Autodesk Inventor part; units mm, degrees
ref_plane "YZ Plane" through (0, 0, 0) normal (1, 0, 0) x (0, 1, 0)
ref_plane "XZ Plane" through (0, 0, 0) normal (0, 1, 0) x (-1, 0, 0)
ref_plane "XY Plane" through (0, 0, 0) normal (0, 0, 1) x (1, 0, 0)
sketch "Sketch1" plane through (0, 0, 0) normal (0, 0, 1) x (1, 0, 0)
  line L0 (0, 0) -> (0, 50)
  line L1 (0, 50) -> (40, 50)
  line L2 (40, 50) -> (40, 20)
  line L3 (40, 20) -> (200, 20)
  line L4 (200, 20) -> (200, 0)
  line L5 (200, 0) -> (0, 0)
  line L6 (20, 50) -> (20, -1.8826)
  line L7 (20, -1.8826) -> (20, 0)
  circle A0 centre (20, 24.0587) radius 10
  dimension "d0" = 200
  dimension "d1" = 50
  dimension "d2" = 40
  dimension "d3" = 20
  dimension "d4" = 20
extrude "Extrusion1" add sketch "Sketch1" along normal blind 140 contours L0 L1 L6 A0 L5 | L6 A0 L1 L2 L3 L4 L5
fillet "Fillet1" radius 15 4 edges at (0, 50, 70) (40, 50, 70) (40, 20, 70) (0, 0, 70)
fillet "Fillet2" radius 20 2 edges at (200, 10, 140) (200, 10, 0)
fillet "Fillet3" radius 4 22 edges at (4.3933, 45.6067, 0) (0, 25, 0) (4.3933, 4.3933, 0) (97.4998, 0, 0) (194.1421, 0, 5.8579) (200, 0, 70) (194.1421, 0, 134.1421) (97.4998, 0, 140) (4.3933, 4.3933, 140) (0, 25, 140) (4.3933, 45.6067, 140) (20, 50, 140) (35.6067, 45.6067, 140) (40, 35, 140) (117.4998, 20, 140) (194.1421, 20, 134.1421) (200, 20, 70) (194.1421, 20, 5.8579) (117.4998, 20, 0) (40, 35, 0) (35.6067, 45.6067, 0) (20, 50, 0)
properties part number "foot rest EG26"
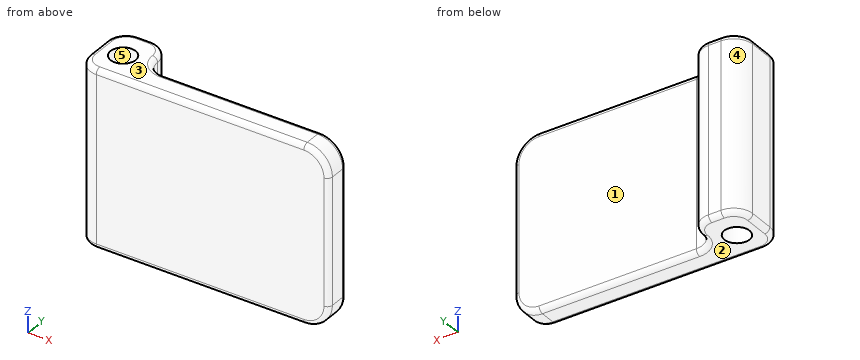
Could you check a few things on this model? Use its own coordinates, in mm. Face numbers are marked on the shaded views. A direction names the side the tool comes from. Coordinates: 2 decimals unless noted, no trailing zeros. Order: outer loops, then holes, each group sorted by start corner. A loop starts at its lowest first (then second) coordinate and runs counter-clockwise, first axis right, second up. Notation, with made-up numbers: (-26, 51) - (-1, 51) arc R20 ccw to (-1, 74) - close; hole circle Ø2 at (19, 1.5). An arc over 180 degrees is marked (long way). Answer in a Markdown table with one row per item. Add a question column.
(1) Will this pin go through, and if not, where does the flat tip stop? pin 1 (4 mm diameter, centred on x = 164, z = 114, fed in from +Y).
(2) If we section it at B-B, the plane x = 100.5: Please give me the cut outline in (y, z), then the cut area to 3 significant figures.
(3) I need wall thicknesses on L1, parallel to Y at x = 20, z = 46; L2, parallel to Y at x = 164, z = 89; L3, parallel to X at y = 15.5, z = 127.5. Which ranges of each line are inside material? Lowest first, please.
(4) If we mould it in two halves opening along Y, with no side actions, what happens to the marked faces 3, 4 and 5? For each: released by +Y, released by -Y, zero draft, split by the parting line, or undercut.
(5) On a 3-axis mill with a long thin cutter (end or side, diameter ignored), from which of +Z, -Z, +X, -X, +Y, -Y can I reach the whole of each face in a straight line? I mean the marked faces 1 and 2. Say none if no direction works.
(6) If we section it at A-A, the plane x = 20: Please give me the cut outline in (y, z).
Results are:
| question | item | result |
|---|---|---|
| 1 | pin 1 | stops at y = 20 |
| 2 | outline | (0, 4) arc R4 ccw to (4, 0) - (16, 0) arc R4 ccw to (20, 4) - (20, 136) arc R4 ccw to (16, 140) - (4, 140) arc R4 ccw to (0, 136) - close |
| 2 | area | 2,790 mm2 |
| 3 | L1 | y = 0 to 14.06, 34.06 to 50 |
| 3 | L2 | y = 0 to 20 |
| 3 | L3 | x = 0 to 14.83, 25.17 to 198.54 |
| 4 | face 3 | zero draft |
| 4 | face 4 | released by +Y |
| 4 | face 5 | undercut |
| 5 | face 1 | +Z, -Z, +X, +Y |
| 5 | face 2 | -Z, +X, -X, +Y, -Y |
| 6 | outline | (0, 4) arc R4 ccw to (4, 0) - (14.06, 0) - (14.06, 140) - (4, 140) arc R4 ccw to (0, 136) - close; (34.06, 0) - (46, 0) arc R4 ccw to (50, 4) - (50, 136) arc R4 ccw to (46, 140) - (34.06, 140) - close |
